```python
from build123d import *

# Parameters (mm, degrees)
SKETCH1_R           = 0.5
SKETCH1_R_2         = 1
BOSS_EXTRUDE1_DEPTH = 0.75
SKETCH2_R           = 3.5
SKETCH2_R_2         = 2.375
BOSS_EXTRUDE2_DEPTH = 3
SKETCH4_R           = 2.6
SKETCH4_R_2         = 2.5
EXTRUDE_THIN1_DEPTH = 0.5
CUT_EXTRUDE1_START  = -0.5
SKETCH5_R           = 2.5
CUT_EXTRUDE1_DEPTH  = 0.5
MOVE_FACE1_BY       = 0.5


with BuildPart() as part:
    # Sketch1 → Boss-Extrude1 (new, symmetric)
    with BuildSketch(Plane(origin=(0, 0, 0), x_dir=(1, 0, 0), z_dir=(0, 1, 0))):
        with BuildLine():
            Line((-2.612867, -2.328718), (-1.996279, -12.421951))
            ThreePointArc((-1.996279, -12.421951), (0, -14.3), (1.996279, -12.421951))
            Line((1.996279, -12.421951), (2.612867, -2.328718))
            ThreePointArc((2.612867, -2.328718), (0, 3.5), (-2.612867, -2.328718))
        make_face()
        with Locations(Location((0, -12.3, 0), (0, 0, 270))):
            Circle(SKETCH1_R, mode=Mode.SUBTRACT)
        with Locations(Location((0, -10.3, 0), (0, 0, 270))):
            Circle(SKETCH1_R, mode=Mode.SUBTRACT)
        with Locations(Location((0, -8.3, 0), (0, 0, 270))):
            Circle(SKETCH1_R, mode=Mode.SUBTRACT)
        with Locations(Location((0, -6.3, 0), (0, 0, 270))):
            Circle(SKETCH1_R, mode=Mode.SUBTRACT)
        with Locations(Location((0, -4.3, 0), (0, 0, 270))):
            Circle(SKETCH1_R, mode=Mode.SUBTRACT)
        with Locations(Location((0, 0, 0), (0, 0, 270))):
            Circle(SKETCH1_R_2, mode=Mode.SUBTRACT)
    extrude(amount=BOSS_EXTRUDE1_DEPTH, both=True)

    # Sketch2 → Boss-Extrude2 (add)
    with BuildSketch(Plane.XZ.offset(0.75)):
        with Locations(Location((0, 0, 0), (0, 0, 270))):
            Circle(SKETCH2_R)
        with Locations(Location((0, 0, 0), (0, 0, 270))):
            Circle(SKETCH2_R_2, mode=Mode.SUBTRACT)
    extrude(amount=BOSS_EXTRUDE2_DEPTH)

    # Sketch4 → Extrude-Thin1 (add)
    with BuildSketch(Plane(origin=(0, 0.75, 0), x_dir=(1, 0, 0), z_dir=(0, 1, 0))):
        Circle(SKETCH4_R)
        Circle(SKETCH4_R_2, mode=Mode.SUBTRACT)
    extrude(amount=EXTRUDE_THIN1_DEPTH)

    # Sketch5 → Cut-Extrude1 (cut)
    with BuildSketch(Plane(origin=(0, 0.75, 0), x_dir=(1, 0, 0), z_dir=(0, 1, 0)).offset(CUT_EXTRUDE1_START)):
        Circle(SKETCH5_R)
    extrude(amount=CUT_EXTRUDE1_DEPTH, mode=Mode.SUBTRACT)

    # Move Face1: a face moved outward by 0.5
    extrude(part.faces().sort_by_distance((0, -0.75, 1.1875))[0], amount=MOVE_FACE1_BY, dir=(0, -1, 0))


solid = part.part
```
Verification items for the finished model (mm, model axes). A direction names the side the tool comes from. Round coordinates to 2 decimals unless told otherwise and drop trailing zeros. Loops run counter-clockwise (first coordinate to the right, second up) from the corner with the lowest first, then second, coordinate; pieces in that order, holes last. Notation, with made-up numbers: (53.25, 57.5) -> (72.25, 57.5) arc R28 cw to (72.25, 82.5) -> close; hole circle Ø3 at (8.25, -23.5). An arc over 180 degrees is marked (long way). Answer as a JSON object with one key per item and string values.
Q1. Section check A-A (z = 0). Record the boundary of the cut face in (x, y) (3 decimals), then the cut area to 3 significant figures.
Data:
{"outline": "(-3.5, -3.75) -> (-2.375, -3.75) -> (-2.375, -1.25) -> (-1, -1.25) -> (-1, 0.25) -> (-2.5, 0.25) -> (-2.5, 1.25) -> (-2.6, 1.25) -> (-2.6, 0.75) -> (-3.5, 0.75) -> close; (1, -1.25) -> (2.375, -1.25) -> (2.375, -3.75) -> (3.5, -3.75) -> (3.5, 0.75) -> (2.6, 0.75) -> (2.6, 1.25) -> (2.5, 1.25) -> (2.5, 0.25) -> (1, 0.25) -> close", "area": "14.2 mm2"}
Q2. Access from +Z, -Z, +X, -X, +Y, -Y to the whole of each face (thin tool, end or side, straight path). Record for faces 1 (the flat face through (1, 0.25, 1)), 2 (the cylindrical face through (-0.444, -0.01, 4.531)), 3 (the cylindrical face through (-1.45, -2.48, 1.88)).
Data:
{"face 1": "+Y", "face 2": "+Y, -Y", "face 3": "-Y"}
Q3. Draft check along Z on faces 4 (the flat face through (1, -0.75, 8)), 5 (the flat face through (2.3, 0.01, 7.45)), 6 (the cylindrical face through (0, 0, 11.8)). Enter one of: pulls with the +Z half, pulls with the -Z half, needs draft (parallel to the pull), parting line crosses it, or undercut.
Data:
{"face 4": "needs draft", "face 5": "pulls with the +Z half", "face 6": "undercut"}
Q4. Go/stop test with flat-tipped pins: P1, Ø3, axis at x = 0, z = 0, coming from the -Y side; P2, Ø2.5, axis at x = 0, z = 0, coming from the +Y side; P3, Ø2, axis at x = 0, z = 11.5, coming from the +Y side; P4, Ø1.8, axis at x = 0, z = 0, coming from the +Y side. Record where each tip stops, or that it passes through.
Data:
{"P1": "stops at y = -1.25", "P2": "stops at y = 0.25", "P3": "stops at y = 0.75", "P4": "passes through"}
Q5. Section check B-B (y = -1.9). Record the boundary of the cut face in (x, z) (3 decimals), then the cut area to 3 significant figures.
Data:
{"outline": "circle Ø7 at (0, 0); hole circle Ø4.75 at (0, 0)", "area": "20.8 mm2"}
Q6. Scan lines: line 1 (X direction, y = -0.3, z = 0); line 2 (X direction, y = -2.2, z = 0) (3 decimals); line 3 (Y direction, x = 0.75, z = 3). Record each from-to range of solid material in increasing order. Write a range as from..to.
Data:
{"line 1": "x = -3.5..-1, 1..3.5", "line 2": "x = -3.5..-2.375, 2.375..3.5", "line 3": "y = -3.75..0.75"}
Q7. Section check C-C (x = 0). State how many separate pieces and enclosed holes the cut face has, then the cut area to 3 significant figures.
Data:
{"separate pieces": "7", "enclosed holes": "0", "area": "22.9 mm2"}
Q8. Section check D-D (z = 4.3). Record the boundary of the cut face in (x, y).
Data:
{"outline": "(-2.49, -0.75) -> (-0.5, -0.75) -> (-0.5, 0.75) -> (-2.49, 0.75) -> close; (0.5, -0.75) -> (2.49, -0.75) -> (2.49, 0.75) -> (0.5, 0.75) -> close"}
